The listing builds one solid part. Answer for the finished solid, in the listing's coordinates (mm). A direction names the side the tool comes from. Give positions to 0.01 mm unless a question says otherwise; leave off trailing zeros. Write each loop counter-clockwise with the first axis right and the second up, starting at its lowest first coordinate (ties: lowest second). Pieces come first, ordered by that corner, then holes. Notation, with made-up numbers: M -1,43.5 L 7,43.5 A21 ccw 7,67.5 Z; hole C 21.25,13.5 d4. An arc over 180 degrees is marked long. Answer as a JSON object with one key per item and string values.
```python
from build123d import *

# Parameters (mm, degrees)
BOSS_EXTRUDE1_DEPTH = 5
SKETCH2_W           = 30
SKETCH2_H           = 70
CUT_EXTRUDE1_DEPTH  = 5
CUT_EXTRUDE2_DEPTH  = 5
SKETCH5_R           = 2.5
SKETCH5_R_2         = 5
CUT_EXTRUDE3_DEPTH  = 5
SKETCH6_R           = 2.5
CUT_EXTRUDE4_DEPTH  = 5
SKETCH7_R           = 12.5
SKETCH7_R_2         = 2.5
CUT_EXTRUDE5_DEPTH  = 5


with BuildPart() as part:
    # Sketch1 → Boss-Extrude1 (new body)
    with BuildSketch(Plane.XY):
        with BuildLine():
            Line((-90, -100), (90, -100))
            ThreePointArc((90, -100), (97.071067812, -97.071067812), (100, -90))
            Line((100, -90), (100, 70))
            ThreePointArc((100, 70), (91.213203436, 91.213203436), (70, 100))
            Line((70, 100), (-70, 100))
            ThreePointArc((-70, 100), (-91.213203436, 91.213203436), (-100, 70))
            Line((-100, 70), (-100, -90))
            ThreePointArc((-100, -90), (-97.071067812, -97.071067812), (-90, -100))
        make_face()
    extrude(amount=BOSS_EXTRUDE1_DEPTH)

    # Sketch2 → Cut-Extrude1 (cut)
    with BuildSketch(Plane.XY.offset(5)):
        with Locations((85, -55)):
            Rectangle(SKETCH2_W, SKETCH2_H)
        with Locations((-85, -55)):
            Rectangle(SKETCH2_W, SKETCH2_H)
    extrude(amount=-CUT_EXTRUDE1_DEPTH, mode=Mode.SUBTRACT)

    # Sketch3 → Cut-Extrude2 (cut)
    with BuildSketch(Plane.XY.offset(5)):
        with BuildLine():
            Line((85, -20), (100, -20))
            Line((100, -20), (100, 70))
            add(Edge.make_bspline(
                [(100, 70), (41.562750789, 76.769648156), (85, -20)],
                knots=[0, 0, 0, 1, 1, 1], degree=2))
        make_face()
        with BuildLine():
            Line((-85, -20), (-100, -20))
            Line((-100, -20), (-100, 70))
            add(Edge.make_bspline(
                [(-100, 70), (-41.562750789, 76.769648156), (-85, -20)],
                knots=[0, 0, 0, 1, 1, 1], degree=2))
        make_face()
    extrude(amount=-CUT_EXTRUDE2_DEPTH, mode=Mode.SUBTRACT)

    # Sketch5 → Cut-Extrude3 (cut)
    with BuildSketch(Plane.XY.offset(5)):
        with Locations((45, -80)):
            Circle(SKETCH5_R)
        with Locations((-45, -80)):
            Circle(SKETCH5_R)
        with Locations(Location((45, -20, 0), (0, 0, 180))):
            Circle(SKETCH5_R)
        with Locations(Location((-45, -20, 0), (0, 0, 180))):
            Circle(SKETCH5_R)
        with Locations((-45, 43.350998567)):
            Circle(SKETCH5_R_2)
        with Locations(Location((45, 43.350998567, 0), (0, 0, 180))):
            Circle(SKETCH5_R_2)
        with Locations((0, -30)):
            Circle(SKETCH5_R)
    extrude(amount=-CUT_EXTRUDE3_DEPTH, mode=Mode.SUBTRACT)

    # Sketch6 → Cut-Extrude4 (cut)
    with BuildSketch(Plane.XY.offset(5)):
        with Locations((0, -90)):
            Circle(SKETCH6_R)
    extrude(amount=-CUT_EXTRUDE4_DEPTH, mode=Mode.SUBTRACT)

    # Sketch7 → Cut-Extrude5 (cut)
    with BuildSketch(Plane(origin=(0, 0, 0), x_dir=(-1, 0, 0), z_dir=(0, 0, -1))):
        with Locations((0, 40)):
            Circle(SKETCH7_R)
        with Locations((-21, 40)):
            Circle(SKETCH7_R_2)
        with Locations((21.26, 40)):
            Circle(SKETCH7_R_2)
    extrude(amount=-CUT_EXTRUDE5_DEPTH, mode=Mode.SUBTRACT)


solid = part.part
```
1. For faces 1 (the flat face through (-85, -90, 3)), 2 (the flat face through (85, -90, 3)), 3 (the flat face through (-1, -100, 2)), determine the directions among +Z, -Z, +X, -X, +Y, -Y from which every point of the face is accessible in a straight line to the end or side of a thin tool.
Verdict:
{"face 1": "+Z, -Z, -X", "face 2": "+Z, -Z, +X", "face 3": "+Z, -Z, +X, -X, -Y"}
2. The mould has two halves that part along Y. Classify faces 4 (the cylindrical face through (96.99, -97.15, 2.46)), 5 (the cylindrical face through (-90.979, 91.445, 2.465)), 6 (the cylindrical face through (-19.276, 38.479, 2.465)), 7 (the cylindrical face through (43.66, -22.11, 2.54)): released by +Y, released by -Y, zero draft, split by the parting line, or undercut.
Verdict:
{"face 4": "released by -Y", "face 5": "released by +Y", "face 6": "undercut", "face 7": "undercut"}
3. A cutting plane is placed at C-C, the plane y = -30. Give the vertices of the cut face in (x, z).
Verdict:
{"outline": "M -70,0 L -2.5,0 L -2.5,5 L -70,5 Z; M 2.5,0 L 70,0 L 70,5 L 2.5,5 Z"}
4. Consider line 1 along Y through (x, z) = (-45, 3.6); line 2 along Y through (x, z) = (0, 1.55); line 3 along Y through (x, z) = (21, 2.4). Determine where each line is inside the solid, lowest interval first.
Verdict:
{"line 1": "y = -100 to -82.5, -77.5 to -22.5, -17.5 to 38.35, 48.35 to 100", "line 2": "y = -100 to -92.5, -87.5 to -32.5, -27.5 to 27.5, 52.5 to 100", "line 3": "y = -100 to 37.5, 42.5 to 100"}
5. A cutting plane is placed at A-A, the plane y = -80. Give the vertices of the cut face in (x, z).
Verdict:
{"outline": "M -70,0 L -47.5,0 L -47.5,5 L -70,5 Z; M -42.5,0 L 42.5,0 L 42.5,5 L -42.5,5 Z; M 47.5,0 L 70,0 L 70,5 L 47.5,5 Z"}
6. A cutting plane is placed at D-D, the plane x = -21.26. Give the vertices of the cut face in (y, z).
Verdict:
{"outline": "M -100,0 L 37.5,0 L 37.5,5 L -100,5 Z; M 42.5,0 L 100,0 L 100,5 L 42.5,5 Z"}
7. A cutting plane is placed at B-B, the plane x = 45. Give the vertices of the cut face in (y, z).
Verdict:
{"outline": "M -100,0 L -82.5,0 L -82.5,5 L -100,5 Z; M -77.5,0 L -22.5,0 L -22.5,5 L -77.5,5 Z; M -17.5,0 L 38.35,0 L 38.35,5 L -17.5,5 Z; M 48.35,0 L 100,0 L 100,5 L 48.35,5 Z"}
8. Flat-ended cylindrical pins translate along their axes: pin 1 (2.5 mm diameter, centred on y = -51, z = 1.5, fed in from -X); pin 2 (1.5 mm diameter, centred on y = 31, z = 3, fed in from -X); pin 3 (1.5 mm diameter, centred on x = 91.5, z = 2, fed in from +Y). Find the tip coordinate at first contact, or state that the pin passes through.
Verdict:
{"pin 1": "stops at x = -70", "pin 2": "stops at x = -67.82", "pin 3": "stops at y = 91.67"}
